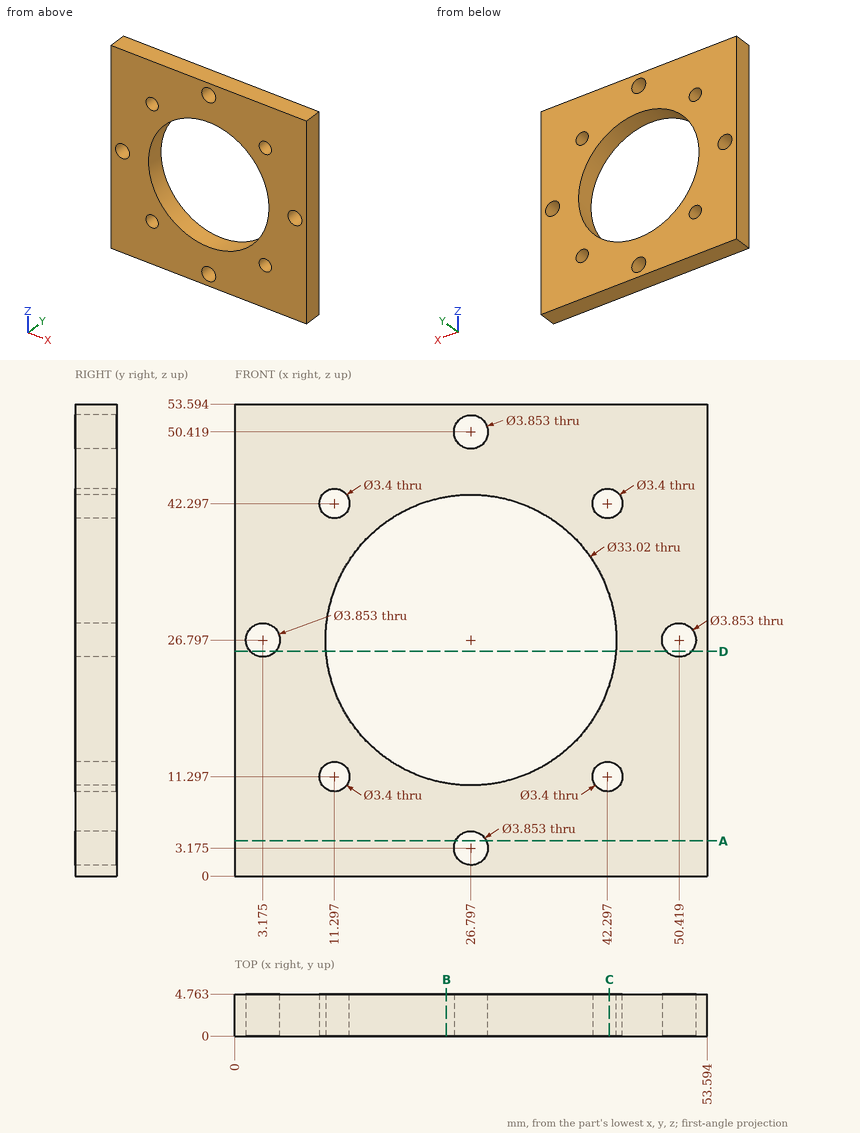
Input: dimensioned drawing with shaded views. Units: mm. Origin: part minimum x, y, z. Give positions to 0.01 mm unless a question says otherwise; leave off trailing zeros. Write each loop counter-clockwise with the first axis right and the second up, starting at its lowest first coordinate (ties: lowest second). Pieces come first, ordered by that corner, then holes. Notation, with made-up numbers: M 29,41.5 L 78,41.5 A27 cw 78,78.5 Z; hole C 3,48.5 d4. An arc over 180 degrees is marked long. Return JSON: item names as keys, results as strings. Group by question number.
1) Cut plane B-B, the plane x = 24. Output: boundary loops of the cut face in (y, z) (1 decimal).
2) Pin query (flat end, axial travel): P1, Ø2, axis at x = 42.297, z = 11.297, coming from the -Y side. Return the tip coordinate at first contact, or that it passes through.
3) Material intervals for line 1 along Z through (x, y) = (41.5, 1.35) (1 decimal); line 2 along X through (y, z) = (3.75, 42) (1 decimal); line 3 along X through (y, z) = (0.65, 10) (1 decimal), sorted ascending. Write a range as [from, to].
4) Cut plane A-A, the plane z = 4. Output: boundary loops of the cut face in (x, y) (1 decimal).
5) Cut plane C-C, the plane x = 42.5. Output: boundary loops of the cut face in (y, z) (1 decimal).
6) Cut plane D-D, the plane z = 25.5. Give the number of separate pieces and of enclosed holes in the cut face.
Recorded:
{
 "1": {"outline": "M 0,0 L 4.8,0 L 4.8,10.5 L 0,10.5 Z; M 0,43.1 L 4.8,43.1 L 4.8,53.6 L 0,53.6 Z"},
 "2": {"P1": "passes through"},
 "3": {"line 1": "z = [0, 9.8], [12.8, 19.3], [34.3, 40.8], [43.8, 53.6]", "line 2": "x = [0, 9.6], [13, 20.4], [33.2, 40.6], [44, 53.6]", "line 3": "x = [0, 10.2], [12.4, 41.2], [43.4, 53.6]"},
 "4": {"outline": "M 0,0 L 25.1,0 L 25.1,4.8 L 0,4.8 Z; M 28.5,0 L 53.6,0 L 53.6,4.8 L 28.5,4.8 Z"},
 "5": {"outline": "M 0,0 L 4.8,0 L 4.8,9.6 L 0,9.6 Z; M 0,13 L 4.8,13 L 4.8,21.7 L 0,21.7 Z; M 0,31.9 L 4.8,31.9 L 4.8,40.6 L 0,40.6 Z; M 0,44 L 4.8,44 L 4.8,53.6 L 0,53.6 Z"},
 "6": {"separate pieces": "4", "enclosed holes": "0"}
}
